Build history of the part. All positions in model axes, mm. A direction names the side the tool comes from. Round coordinates to 2 decimals unless told otherwise and drop trailing zeros. Order: outer loops, then holes, each group sorted by start corner. A loop starts at its lowest first (then second) coordinate and runs counter-clockwise, first axis right, second up. Notation, with made-up numbers: M 61.25,72 L 76.25,72 A17 ccw 76.25,90 Z; hole C 63.25,61.5 d6. An arc over 180 degrees is marked long. Use CSV: the item, a comma, the result in double quotes.
from build123d import *

# Parameters (mm, degrees)
SKETCH1_W                      = 20
SKETCH1_H                      = 60
BASE_FLANGE1_DEPTH             = 2
EDGE_FLANGE1_STRIP_CUT_DEPTH   = 20
EDGE_FLANGE1_DEPTH             = 20
EDGE_FLANGE2_STRIP_CUT_DEPTH   = 20
EDGE_FLANGE2_DEPTH             = 20
EDGE_FLANGE3_STRIP_CUT_DEPTH   = 20
EDGE_FLANGE3_DEPTH             = 20
EDGE_FLANGE3_START             = 2
EDGE_FLANGE3_FLAT_DEPTH        = 2
EDGE_FLANGE4_STRIP_CUT_DEPTH   = 20
EDGE_FLANGE4_STRIP_CUT_2_DEPTH = 20
EDGE_FLANGE4_DEPTH             = 20
EDGE_FLANGE4_BEND_DEPTH        = 20
SKETCH16_W                     = 5
SKETCH16_H                     = 15
CUT_EXTRUDE2_DEPTH             = 142.77897769
SKETCH23_R                     = 4
SKETCH23_R_2                   = 1.5
CUT_EXTRUDE3_DEPTH             = 2


# Sheet-metal steps are written as plain solids
with BuildPart() as part:
    # Sketch1 → Base-Flange1 (new body)
    with BuildSketch(Plane.XY):
        Rectangle(SKETCH1_W, SKETCH1_H)
    extrude(amount=-BASE_FLANGE1_DEPTH)

    # Edge-Flange1 strip (across the edge) → Edge-Flange1 strip cut (cut)
    with BuildSketch(Plane(origin=(-10, 30, -2), x_dir=(0, -0.3420201433256631, -0.9396926207859105), z_dir=(1, 0, 0))):
        Polygon((-5.074988048, 8.095806265), (-1.834962826, -0.80608987), (0.044422416, -0.122049584), (-3.195602806, 8.779846552), align=None)
    extrude(amount=EDGE_FLANGE1_STRIP_CUT_DEPTH, mode=Mode.SUBTRACT)

    # Edge-Flange1 section (across the edge) → Edge-Flange1 (add)
    with BuildSketch(Plane(origin=(-10, 30, -2), x_dir=(0, -0.3420201433256631, -0.9396926207859105), z_dir=(1, 0, 0))):
        with BuildLine():
            Line((-2, 0.129882454), (-2, 39.647346039))
            Line((-2, 39.647346039), (0, 39.647346039))
            Line((0, 39.647346039), (0, 0.129882454))
            ThreePointArc((0, 0.129882454), (0.011190609, 0.001973206), (0.044422416, -0.122049584))
            Line((0.044422416, -0.122049584), (-1.834962826, -0.80608987))
            ThreePointArc((-1.834962826, -0.80608987), (-1.958424897, -0.345323149), (-2, 0.129882454))
        make_face()
    extrude(amount=EDGE_FLANGE1_DEPTH)

    # Edge-Flange2 strip (across the edge) → Edge-Flange2 strip cut (cut)
    with BuildSketch(Plane(origin=(10, -30, -2), x_dir=(0, 0.34202014332566344, -0.9396926207859103), z_dir=(-1, 0, 0))):
        Polygon((-5.074988048, 8.095806265), (-1.834962826, -0.80608987), (0.044422416, -0.122049584), (-3.195602806, 8.779846552), align=None)
    extrude(amount=EDGE_FLANGE2_STRIP_CUT_DEPTH, mode=Mode.SUBTRACT)

    # Edge-Flange2 section (across the edge) → Edge-Flange2 (add)
    with BuildSketch(Plane(origin=(10, -30, -2), x_dir=(0, 0.34202014332566344, -0.9396926207859103), z_dir=(-1, 0, 0))):
        with BuildLine():
            Line((-2, 0.129882454), (-2, 49.647346039))
            Line((-2, 49.647346039), (0, 49.647346039))
            Line((0, 49.647346039), (0, 0.129882454))
            ThreePointArc((0, 0.129882454), (0.011190609, 0.001973206), (0.044422416, -0.122049584))
            Line((0.044422416, -0.122049584), (-1.834962826, -0.80608987))
            ThreePointArc((-1.834962826, -0.80608987), (-1.958424897, -0.345323149), (-2, 0.129882454))
        make_face()
    extrude(amount=EDGE_FLANGE2_DEPTH)

    # Edge-Flange3 strip (across the edge) → Edge-Flange3 strip cut (cut)
    with BuildSketch(Plane(origin=(-10, 67.256318506, -15.560190975), x_dir=(0, -0.6427876096865303, -0.7660444431189858), z_dir=(1, 0, 0))):
        Polygon((-5.074988048, 8.095806265), (-1.834962826, -0.80608987), (0.044422416, -0.122049584), (-3.195602806, 8.779846552), align=None)
    extrude(amount=EDGE_FLANGE3_STRIP_CUT_DEPTH, mode=Mode.SUBTRACT)

    # Edge-Flange3 bend section (across the edge) → Edge-Flange3 (add)
    with BuildSketch(Plane(origin=(-10, 67.256318506, -15.560190975), x_dir=(0, -0.6427876096865303, -0.7660444431189858), z_dir=(1, 0, 0))):
        with BuildLine():
            Line((-2, 0.129882454), (0, 0.129882454))
            ThreePointArc((0, 0.129882454), (0.011190609, 0.001973206), (0.044422416, -0.122049584))
            Line((0.044422416, -0.122049584), (-1.834962826, -0.80608987))
            ThreePointArc((-1.834962826, -0.80608987), (-1.958424897, -0.345323149), (-2, 0.129882454))
        make_face()
    extrude(amount=EDGE_FLANGE3_DEPTH)

    # Edge-Flange3 profile (on flange) → Edge-Flange3 flat (add)
    with BuildSketch(Plane(origin=(0, 67.256318506, -15.560190975), x_dir=(1, 0, 0), z_dir=(0, 0.6427876096865303, 0.7660444431189858)).offset(EDGE_FLANGE3_START)):
        Polygon((10, 0.129882454), (10, 19.823673019), (27.5, 19.823673019), (27.5, 39.823673019), (10, 39.823673019), (10, 59.647346039), (-10, 59.647346039), (-10, 39.823673019), (-27.5, 39.823673019), (-27.5, 19.823673019), (-10, 19.823673019), (-10, 0.129882454), align=None)
    extrude(amount=-EDGE_FLANGE3_FLAT_DEPTH)

    # Edge-Flange4 strip (across the edge) → Edge-Flange4 strip cut (cut)
    with BuildSketch(Plane(origin=(27.5, 97.763021927, -41.158354564), x_dir=(-0.34202014332566383, -0.6040227735550463, -0.7198463103929629), z_dir=(0, -0.7660444431189858, 0.6427876096865304))):
        Polygon((-5.074988048, 8.095806265), (-1.834962826, -0.80608987), (0.044422416, -0.122049584), (-3.195602806, 8.779846552), align=None)
    extrude(amount=EDGE_FLANGE4_STRIP_CUT_DEPTH, mode=Mode.SUBTRACT)

    # Edge-Flange4 strip 2 (across the edge) → Edge-Flange4 strip cut 2 (cut)
    with BuildSketch(Plane(origin=(-27.5, 82.442133065, -28.30260237), x_dir=(0.3420201433256639, -0.6040227735550463, -0.7198463103929628), z_dir=(0, 0.7660444431189859, -0.6427876096865303))):
        Polygon((-5.074988048, 8.095806265), (-1.834962826, -0.80608987), (0.044422416, -0.122049584), (-3.195602806, 8.779846552), align=None)
    extrude(amount=EDGE_FLANGE4_STRIP_CUT_2_DEPTH, mode=Mode.SUBTRACT)

    # Edge-Flange4 section (across the edge) → Edge-Flange4 (add)
    with BuildSketch(Plane(origin=(27.5, 97.763021927, -41.158354564), x_dir=(-0.34202014332566383, -0.6040227735550463, -0.7198463103929629), z_dir=(0, -0.7660444431189858, 0.6427876096865304))):
        with BuildLine():
            Line((-2, 0.129882454), (-2, 19.647346039))
            Line((-2, 19.647346039), (0, 19.647346039))
            Line((0, 19.647346039), (0, 0.129882454))
            ThreePointArc((0, 0.129882454), (0.011190609, 0.001973206), (0.044422416, -0.122049584))
            Line((0.044422416, -0.122049584), (-1.834962826, -0.80608987))
            ThreePointArc((-1.834962826, -0.80608987), (-1.958424897, -0.345323149), (-2, 0.129882454))
        make_face()
    extrude(amount=EDGE_FLANGE4_DEPTH)

    # Edge-Flange4 section 2 (across the edge) → Edge-Flange4 bend (add)
    with BuildSketch(Plane(origin=(-27.5, 82.442133065, -28.30260237), x_dir=(0.3420201433256639, -0.6040227735550463, -0.7198463103929628), z_dir=(0, 0.7660444431189859, -0.6427876096865303))):
        with BuildLine():
            Line((-2, 0.129882454), (-2, 19.647346039))
            Line((-2, 19.647346039), (0, 19.647346039))
            Line((0, 19.647346039), (0, 0.129882454))
            ThreePointArc((0, 0.129882454), (0.011190609, 0.001973206), (0.044422416, -0.122049584))
            Line((0.044422416, -0.122049584), (-1.834962826, -0.80608987))
            ThreePointArc((-1.834962826, -0.80608987), (-1.958424897, -0.345323149), (-2, 0.129882454))
        make_face()
    extrude(amount=EDGE_FLANGE4_BEND_DEPTH)

    # Sketch16 → Cut-Extrude2 (cut, through all)
    with BuildSketch(Plane(origin=(0, -3.55058603, 9.755154944), x_dir=(1, 0, 0), z_dir=(0, -0.3420201433256634, 0.9396926207859103))):
        with Locations((-7.5, -71.022164949)):
            Rectangle(SKETCH16_W, SKETCH16_H)
        with Locations((7.5, -71.022164949)):
            Rectangle(SKETCH16_W, SKETCH16_H)
    extrude(amount=-CUT_EXTRUDE2_DEPTH, mode=Mode.SUBTRACT)

    # Sketch23 → Cut-Extrude3 (cut)
    with BuildSketch(Plane(origin=(0, 20.126792325, 23.986177061), x_dir=(-1, 0, 0), z_dir=(0, -0.6427876096865301, -0.7660444431189858))):
        with Locations(Location((0, 102.346900038, 0), (0, 0, 90))):
            Circle(SKETCH23_R)
        with Locations(Location((0, 109.346900038, 0), (0, 0, 90))):
            Circle(SKETCH23_R_2)
        with Locations(Location((7, 102.346900038, 0), (0, 0, 90))):
            Circle(SKETCH23_R_2)
        with Locations(Location((0, 95.346900038, 0), (0, 0, 90))):
            Circle(SKETCH23_R_2)
        with Locations(Location((-7, 102.346900038, 0), (0, 0, 90))):
            Circle(SKETCH23_R_2)
        with Locations(Location((-7, 80.346900038, 0), (0, 0, 270))):
            Circle(SKETCH23_R_2)
        with Locations(Location((7, 80.346900038, 0), (0, 0, 270))):
            Circle(SKETCH23_R_2)
        with Locations(Location((0, 80.346900038, 0), (0, 0, 270))):
            Circle(SKETCH23_R)
        with Locations(Location((0, 87.346900038, 0), (0, 0, 270))):
            Circle(SKETCH23_R_2)
        with Locations(Location((0, 73.346900038, 0), (0, 0, 270))):
            Circle(SKETCH23_R_2)
    extrude(amount=-CUT_EXTRUDE3_DEPTH, mode=Mode.SUBTRACT)


solid = part.part
(1) Drop flat-ended pins along their axis: pin 1 (10 mm diameter, centred on x = -13.5, z = -33, fed in from +Y); pin 2 (7 mm diameter, centred on y = 102.5, z = -44, fed in from -X); pin 3 (7.5 mm diameter, centred on y = -69.5, z = -15, fed in from +X). Give the stop position or say it passes through.
Answer block:
pin 1,"stops at y = 97.11"
pin 2,"stops at x = -10"
pin 3,"stops at x = 5"
(2) Wall check: line 1 (X direction, y = -35.5, z = -2); line 2 (Z direction, x = 2.5, y = -32); line 3 (Y direction, x = -42, z = -37). Give the ranges that are in metal, low to high. Write a range as from..to.
Answer block:
line 1,"x = -10..10"
line 2,"z = -2.73..-0.6"
line 3,"y = 84.6..87.91"
(3) Tool access for faces 1 (the face through (-0.07, 88.82, -32.37)), 2 (the face through (36.92, 88.01, -37.45)), 3 (the face through (0, 0, -2)): list every direction of +Z, -Z, +X, -X, +Y, -Y with a clear straight run to the whole face (end or side of a thin tool).
Answer block:
face 1,"none"
face 2,"-Z, -Y"
face 3,"-Z, +X, -X"
(4) Cut at A-A, the plane y = 21. Give the cut face in (x, z).
Answer block:
outline,"M -10,-2 L 10,-2 L 10,0 L -10,0 Z"
(5) Two-plate mould, pull along Y, no slides. Class faces 4 (the face through (-27.839, 91.255, -33.139)), 5 (the face through (28.987, 82.539, -28.187)), 6 (the face through (0.57, 75.89, -21.51)): released by +Y, released by -Y, zero draft, split by the parting line, or undercut.
Answer block:
face 4,"released by +Y"
face 5,"released by -Y"
face 6,"undercut"
(6) Cut at B-B, the plane x = 12.5. Give the cut face in (y, z).
Answer block:
outline,"M 82.44,-28.3 L 97.76,-41.16 L 99.05,-39.63 L 83.73,-26.77 Z"
